from build123d import *

# Parameters (mm, degrees)
F0_R      = 55
F1_DEPTH  = 50
F2_R      = 75
F3_DEPTH  = 10
F4_R      = 48.288599
F5_DEPTH  = 50
F6_R      = 55.291739
F7_DEPTH  = 50
F8_R      = 39.467294
F9_DEPTH  = 10
F10_R     = 7.5
F11_DEPTH = 50
F12_R     = 28.99692
F13_DEPTH = 25


with BuildPart() as f1:
    # F0 (on Top) → F1 (new body)
    with BuildSketch(Plane.XY):
        Circle(F0_R)
    extrude(amount=F1_DEPTH)

    # F2 (on face) → F3 (join)
    with BuildSketch(Plane.XY.offset(50)):
        Circle(F2_R)
    extrude(amount=F3_DEPTH)

    # F4 (on face) → F5 (join)
    with BuildSketch(Plane(origin=(0, 0, 0), x_dir=(1, 0, 0), z_dir=(0, 0, -1))):
        Circle(F4_R)
    extrude(amount=F5_DEPTH)

    # F6 (on face) → F7 (join)
    with BuildSketch(Plane(origin=(0, 0, -50), x_dir=(1, 0, 0), z_dir=(0, 0, -1))):
        Circle(F6_R)
    extrude(amount=F7_DEPTH)

    # F8 (on face) → F9 (cut)
    with BuildSketch(Plane.XY.offset(60)):
        Circle(F8_R)
    extrude(amount=-F9_DEPTH, mode=Mode.SUBTRACT)

    # F10 (on face) → F11 (join)
    with BuildSketch(Plane.XY.offset(50)):
        Circle(F10_R)
    extrude(amount=F11_DEPTH)

    # F12 (on face) → F13 (join)
    with BuildSketch(Plane(origin=(0, 0, -100), x_dir=(1, 0, 0), z_dir=(0, 0, -1))):
        Circle(F12_R)
    extrude(amount=F13_DEPTH)


solid = f1.part
Work out the finished part from the listing and answer in its coordinate system (mm). A direction names the side the tool comes from. Round coordinates to 2 decimals unless told otherwise and drop trailing zeros. Loops run counter-clockwise (first coordinate to the right, second up) from the corner with the lowest first, then second, coordinate; pieces in that order, holes last. Notation, with made-up numbers: (33.5, -7.5) - (63.5, -7.5) arc R17 ccw to (63.5, 10.5) - close; hole circle Ø2 at (45.5, 40). An arc over 180 degrees is marked (long way). One line per item, written item: value.
Q1. Find section D-D on z = -91. Give the vertices of the cut face in (x, y), and give its area (3 significant figures).
Check values:
outline: circle Ø110.58 at (0, 0)
area: 9,600 mm2
Q2. Straight lines are drawn through the part: probe 1 along Y at (x, z) = (0, 55); probe 2 along Z at (x, y) = (19.5, -64.5); probe 3 along Z at (x, y) = (-27.5, -29.5). For each, find the intervals that lie inside material, in ascending order.
Check values:
probe 1: -75 to -39.47, -7.5 to 7.5, 39.47 to 75
probe 2: 50 to 60
probe 3: -100 to 60
Q3. Find section C-C on z = 84.5. Give the vertices of the cut face in (x, y).
Check values:
outline: circle Ø15 at (0, 0)
Q4. Find section A-A on y = 0. Give the vertices of the cut face in (x, z), and give its area (3 significant figures).
Check values:
outline: (-75, 50) - (-55, 50) - (-55, 0) - (-48.29, 0) - (-48.29, -50) - (-55.29, -50) - (-55.29, -100) - (-29, -100) - (-29, -125) - (29, -125) - (29, -100) - (55.29, -100) - (55.29, -50) - (48.29, -50) - (48.29, 0) - (55, 0) - (55, 50) - (75, 50) - (75, 60) - (39.47, 60) - (39.47, 50) - (7.5, 50) - (7.5, 100) - (-7.5, 100) - (-7.5, 50) - (-39.47, 50) - (-39.47, 60) - (-75, 60) - close
area: 18,800 mm2
Q5. For faces 1 (the flat face through (-1, -8, 50)), 2 (the flat face through (0, 0, -125)), 3 (the cylindrical face through (-28.97, -1.27, -112.32)), 4 (the cylindrical face through (-9.764, 74.362, 54.93)), 5 (the cylindrical face through (46.06, -14.5, -24.65)), determine the directions among +Z, -Z, +X, -X, +Y, -Y from which every point of the face is accessible in a straight line to the end or side of a thin tool.
Check values:
face 1: +Z
face 2: -Z, +X, -X, +Y, -Y
face 3: -Z
face 4: +Z, -Z
face 5: none
Q6. Each of these flat-tipped pins is pushed along its axis until it touches: pin 1 Ø1.5 at (x, y) = (24, -25.5) entering from -Z; pin 2 Ø1 at (y, z) = (-41.5, -6.5) entering from -X; pin 3 Ø10 at (x, z) = (-28.5, 30.5) entering from -Y. Where does it stop, or does it pass through?
Check values:
pin 1: z = -100
pin 2: x = -25.51
pin 3: y = -49.73
Q7. The mould has two halves that part along Z. Classify faces 6 (the flat face through (0, 0, 100)), 7 (the cylindrical face through (-11.923, -53.692, 24.65)), 8 (the flat face through (0, -49, 0)), 9 (the cylindrical face through (-43.88, 33.64, -74.65)): +Z half, -Z half, draft (parallel to the pull), parting line (faces both ways), or undercut.
Check values:
face 6: +Z half
face 7: undercut
face 8: undercut
face 9: draft
